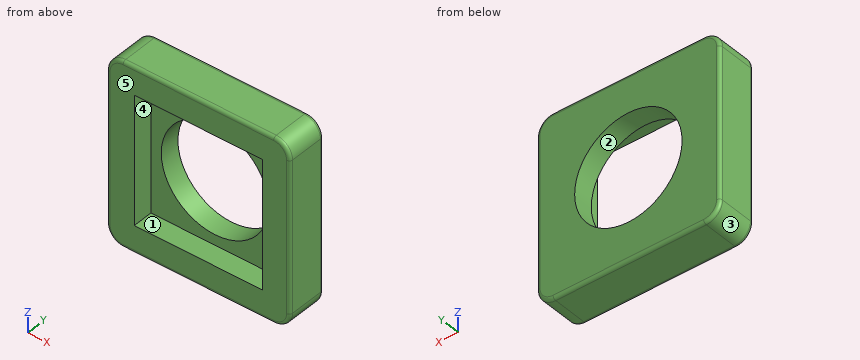
from build123d import *

# Parameters (mm, degrees)
SKETCH1_W           = 57.15
SKETCH1_H           = 57.15
BOSS_EXTRUDE2_DEPTH = 12.7
FILLET1_R           = 5.08
FILLET2_R           = 1.016
SKETCH15_R          = 16.764
CUT_EXTRUDE1_DEPTH  = 6.35
SKETCH16_W          = 40
SKETCH16_H          = 40
CUT_EXTRUDE2_DEPTH  = 6.35


with BuildPart() as part:
    # Sketch1 → Boss-Extrude2 (new body)
    with BuildSketch(Plane(origin=(0, 0, 0), x_dir=(1, 0, 0), z_dir=(0, 1, 0))):
        Rectangle(SKETCH1_W, SKETCH1_H)
    extrude(amount=BOSS_EXTRUDE2_DEPTH)

    # Fillet1
    fillet1_edges = [part.edges().sort_by_distance(p)[0] for p in [
        (28.575, 6.35, 28.575),
        (-28.575, 6.35, 28.575),
        (-28.575, 6.35, -28.575),
        (28.575, 6.35, -28.575),
    ]]
    fillet(fillet1_edges, radius=FILLET1_R)

    # Fillet2
    fillet2_edges = [part.edges().sort_by_distance(p)[0] for p in [
        (0, 0, 28.575),
        (0, 12.7, 28.575),
        (28.575, 0, 0),
        (-28.575, 0, 0),
        (0, 0, -28.575),
        (-27.087102448, 0, -27.087102448),
        (27.087102448, 0, -27.087102448),
        (27.087102448, 0, 27.087102448),
        (-27.087102448, 0, 27.087102448),
        (-28.575, 12.7, 0),
        (28.575, 12.7, 0),
        (0, 12.7, -28.575),
        (-27.087102448, 12.7, -27.087102448),
        (27.087102448, 12.7, -27.087102448),
        (27.087102448, 12.7, 27.087102448),
        (-27.087102448, 12.7, 27.087102448),
    ]]
    fillet(fillet2_edges, radius=FILLET2_R)

    # Sketch15 → Cut-Extrude1 (cut)
    with BuildSketch(Plane(origin=(0, 12.7, 0), x_dir=(1, 0, 0), z_dir=(0, 1, 0))):
        with Locations(Location((0, 0, 0), (0, 0, 270))):
            Circle(SKETCH15_R)
    extrude(amount=-CUT_EXTRUDE1_DEPTH, mode=Mode.SUBTRACT)

    # Sketch16 → Cut-Extrude2 (cut)
    with BuildSketch(Plane.XZ):
        Rectangle(SKETCH16_W, SKETCH16_H)
    extrude(amount=-CUT_EXTRUDE2_DEPTH, mode=Mode.SUBTRACT)


solid = part.part
Build history of the part. All positions in model axes, mm. Face numbers are marked on the shaded views. A direction names the side the tool comes from. Give positions to 0.01 mm unless a question says otherwise; leave off trailing zeros. Order: outer loops, then holes, each group sorted by start corner. A loop starts at its lowest first (then second) coordinate and runs counter-clockwise, first axis right, second up. Notation, with made-up numbers: M 58,36 L 74,36 A20 cw 74,44 Z; hole C 43.25,44 d4. An arc over 180 degrees is marked long. Put each result on its own line as item: value.
Item 1: Cut at C-C on x = 0. Write the cut outline in (y, z) (3 decimals).
Results are:
outline: M 0,-27.559 A1.016 ccw 1.016,-28.575 L 11.684,-28.575 A1.016 ccw 12.7,-27.559 L 12.7,-16.764 L 6.35,-16.764 L 6.35,-20 L 0,-20 Z; M 0,20 L 6.35,20 L 6.35,16.764 L 12.7,16.764 L 12.7,27.559 A1.016 ccw 11.684,28.575 L 1.016,28.575 A1.016 ccw 0,27.559 Z
Item 2: Pull direction X, two halves, no side cores. Call the marked faces 3, 4 and 5: +X half, -X half, draft (parallel to the pull), parting line (faces both ways), or undercut.
Results are:
face 3: -X half
face 4: undercut
face 5: draft
Item 3: Cut at D-D on x = 19. Write the cut outline in (y, z) (3 decimals).
Results are:
outline: M 0,-27.559 A1.016 ccw 1.016,-28.575 L 11.684,-28.575 A1.016 ccw 12.7,-27.559 L 12.7,27.559 A1.016 ccw 11.684,28.575 L 1.016,28.575 A1.016 ccw 0,27.559 L 0,20 L 6.35,20 L 6.35,-20 L 0,-20 Z
Item 4: Cut at B-B on z = 0. Write the cut outline in (x, y) (3 decimals).
Results are:
outline: M -28.575,1.016 A1.016 ccw -27.559,0 L -20,0 L -20,6.35 L -16.764,6.35 L -16.764,12.7 L -27.559,12.7 A1.016 ccw -28.575,11.684 Z; M 16.764,6.35 L 20,6.35 L 20,0 L 27.559,0 A1.016 ccw 28.575,1.016 L 28.575,11.684 A1.016 ccw 27.559,12.7 L 16.764,12.7 Z
Item 5: Which spindle directions (+Z, -Z, +X, -X, +Y, -Y) get a long thin tool onto all of the face, cutting with end or side? Do the marked faces 1 and 2. Say none if no direction does.
Results are:
face 1: -Y
face 2: +Y, -Y
Item 6: Wall check: probe 1 along X at (y, z) = (11.5, 0) (3 decimals); probe 2 along Z at (x, y) = (-10.5, 5.5) (3 decimals). Give the ranges that are in metal, low to high.
Results are:
probe 1: -28.575 to -16.764, 16.764 to 28.575
probe 2: -28.575 to -20, 20 to 28.575
Item 7: Cut at A-A on y = 9.5. Write the cut outline in (x, z) (3 decimals), then the cut area to 3 significant figures.
Results are:
outline: M -28.575,-23.495 A5.08 ccw -23.495,-28.575 L 23.495,-28.575 A5.08 ccw 28.575,-23.495 L 28.575,23.495 A5.08 ccw 23.495,28.575 L -23.495,28.575 A5.08 ccw -28.575,23.495 Z; hole C 0,0 d33.528
area: 2,360 mm2
